Can you work these out from the model? Positions are in its coordinate system, mm. A direction names the side the tool comes from. Give positions to 0.01 mm unless a question says otherwise; leave off trailing zeros. Loops run counter-clockwise (first coordinate to the right, second up) from the corner with the lowest first, then second, coordinate; pieces in that order, holes last. Notation, with made-up numbers: (10, 76.25) - (16, 76.25) arc R7 cw to (16, 84.25) - close; hole circle Ø6 at (-34, 49.5). An arc over 180 degrees is marked (long way). Use a Markdown table: item, result. Add a question column.
```python
from build123d import *

# Parameters (mm, degrees)
SKETCH1_R           = 29
BOSS_EXTRUDE1_DEPTH = 5
CUT_EXTRUDE3_START  = -10
CUT_EXTRUDE3_DEPTH  = 10
FILLET2_R           = 15
FILLET3_R           = 10
SKETCH7_W           = 5
SKETCH7_H           = 5
SKETCH7_W_2         = 7
CUT_EXTRUDE4_DEPTH  = 10


with BuildPart() as part:
    # Sketch1 → Boss-Extrude1 (new body)
    with BuildSketch(Plane.XY):
        Circle(SKETCH1_R)
    extrude(amount=BOSS_EXTRUDE1_DEPTH)

    # Sketch6 → Cut-Extrude3 (cut)
    with BuildSketch(Plane.XY.offset(5).offset(CUT_EXTRUDE3_START)):
        with BuildLine():
            Line((-15.004747761, 24.816477281), (-15.004747761, -24.816477281))
            ThreePointArc((-15.004747761, -24.816477281), (-29, 0), (-15.004747761, 24.816477281))
        make_face()
        with BuildLine():
            Line((14.995252239, 24.822216063), (14.995252239, -24.822216063))
            ThreePointArc((14.995252239, -24.822216063), (29, 0), (14.995252239, 24.822216063))
        make_face()
    extrude(amount=CUT_EXTRUDE3_DEPTH, mode=Mode.SUBTRACT)

    # Fillet2
    fillet2_edges = [part.edges().sort_by_distance(p)[0] for p in [
        (-15.004747761, 24.816477281, 2.5),
        (14.995252239, 24.822216063, 2.5),
    ]]
    fillet(fillet2_edges, radius=FILLET2_R - 0.0001)  # a hair under: the kernel refuses the full size

    # Fillet3
    fillet3_edges = [part.edges().sort_by_distance(p)[0] for p in [
        (-15.004747761, -24.816477281, 2.5),
        (14.995252239, -24.822216063, 2.5),
    ]]
    fillet(fillet3_edges, radius=FILLET3_R)

    # Sketch7 → Cut-Extrude4 (cut)
    with BuildSketch(Plane.XY.offset(5)):
        with Locations((0, 22.499998332)):
            Rectangle(SKETCH7_W, SKETCH7_H)
        with Locations((0, -25.000001668)):
            Rectangle(SKETCH7_W_2, SKETCH7_H)
    extrude(amount=-CUT_EXTRUDE4_DEPTH, mode=Mode.SUBTRACT)


solid = part.part
```
1. On a 3-axis mill with a long thin cutter (end or side, diameter ignored), from which of +Z, -Z, +X, -X, +Y, -Y can I reach the whole of each face in a straight line? I mean faces 1 (the face through (0, -22.5, 3)), 2 (the face through (-15.005, -2, 2)). Say none if no direction works.
2. Suppose I cut it at B-B (z = 2.8). State how many separate pieces and enclosed holes the cut face has, and give its area (3 significant figures).
3. Suppose I cut it at C-C (x = 12.5). List the corners of the cut face in (y, z) for me, and give its area (3 significant figures).
4. Will these pins go through, and if not, where does the flat tip stop? P1, Ø2.5, axis at x = 1.5, z = 2.5, coming from the +Y side; P2, Ø2, axis at x = -8, z = 2.5, coming from the +Y side; P3, Ø1, axis at x = 2, y = 4, coming from the -Z side; P4, Ø3, axis at y = -20.5, z = 3, coming from the -X side.
5. Please list where these lines run through material, in increasing order: line 1 along Y through (x, z) = (0, 1.55); line 2 along X through (y, z) = (23, 3.85); line 3 along Y through (x, z) = (-3, 1.6). Write a range as [from, to].
6. Suppose I cut it at A-A (y = 23). List the corners of the cut face in (x, z) for me.
7. If we mould it in two halves opening along Y, with no side actions, what happens to faces 3 (the face through (0, 0, 0)), 4 (the face through (2.5, 22, 3)), 5 (the face through (-12.897, -24.47, 2.535))? For each: released by +Y, released by -Y, zero draft, split by the parting line, or undercut.
8. Suppose I cut it at D-D (y = -21). List the corners of the cut face in (x, z) for me.
Results below:
| question | item | result |
|---|---|---|
| 1 | face 1 | +Z, -Z |
| 1 | face 2 | +Z, -Z, -X, +Y, -Y |
| 2 | separate pieces | 1 |
| 2 | enclosed holes | 2 |
| 2 | area | 1,530 mm² |
| 3 | outline | (-24.94, 0) - (22.28, 0) - (22.28, 5) - (-24.94, 5) - close |
| 3 | area | 236 mm² |
| 4 | P1 | y = 29 |
| 4 | P2 | y = 27.27 |
| 4 | P3 | z = 0 |
| 4 | P4 | x = -14.98 |
| 5 | line 1 | [-29, -27.5], [-22.5, 20], [25, 29] |
| 5 | line 2 | [-12, -2.5], [2.5, 12] |
| 5 | line 3 | [-28.84, -27.5], [-22.5, 28.7] |
| 6 | outline | (-12, 0) - (-2.5, 0) - (-2.5, 5) - (-12, 5) - close; (2.5, 0) - (12, 0) - (12, 5) - (2.5, 5) - close |
| 7 | face 3 | zero draft |
| 7 | face 4 | undercut |
| 7 | face 5 | released by -Y |
| 8 | outline | (-14.64, 0) - (14.63, 0) - (14.63, 5) - (-14.64, 5) - close |
